Read the model definition and answer for the solid it produces. Units are mm, in the model's axes. Face numbers are marked on the shaded views. Round coordinates to 2 decimals unless told otherwise and drop trailing zeros. Write each loop counter-clockwise with the first axis right and the second up, starting at its lowest first coordinate (ties: lowest second). Pieces come first, ordered by that corner, then holes. Notation, with made-up numbers: (59, 88) -> (66, 88) arc R18 ccw to (66, 118) -> close; hole circle Ø4 at (2, -6.75). An arc over 180 degrees is marked (long way). Return JSON: item names as keys, results as strings.
from build123d import *

# Parameters (mm, degrees)
SKETCH1_W           = 80
SKETCH1_H           = 12
BOSS_EXTRUDE1_DEPTH = 8
SKETCH2_R           = 3
SKETCH2_R_2         = 1
CUT_EXTRUDE1_DEPTH  = 42.231056256
FILLET1_R           = 2


with BuildPart() as part:
    # Sketch1 → Boss-Extrude1 (new body)
    with BuildSketch(Plane(origin=(0, 0, 0), x_dir=(1, 0, 0), z_dir=(0, 1, 0))):
        Rectangle(SKETCH1_W, SKETCH1_H)
    extrude(amount=BOSS_EXTRUDE1_DEPTH)

    # Sketch2 → Cut-Extrude1 (cut, through all)
    with BuildSketch(Plane(origin=(0, 8, 0), x_dir=(1, 0, 0), z_dir=(0, 1, 0))):
        with Locations(Location((-32, 0, 0), (0, 0, 270))):
            Circle(SKETCH2_R)
        with Locations(Location((-12, 0, 0), (0, 0, 270))):
            Circle(SKETCH2_R)
        with Locations(Location((21.25, 0, 0), (0, 0, 270))):
            Circle(SKETCH2_R_2)
        with Locations(Location((30.75, 0, 0), (0, 0, 270))):
            Circle(SKETCH2_R_2)
    extrude(amount=-CUT_EXTRUDE1_DEPTH, mode=Mode.SUBTRACT)

    # Fillet1
    fillet1_edges = [part.edges().sort_by_distance(p)[0] for p in [
        (40, 4, 6),
        (-40, 4, 6),
        (-40, 4, -6),
        (40, 4, -6),
    ]]
    fillet(fillet1_edges, radius=FILLET1_R)


solid = part.part
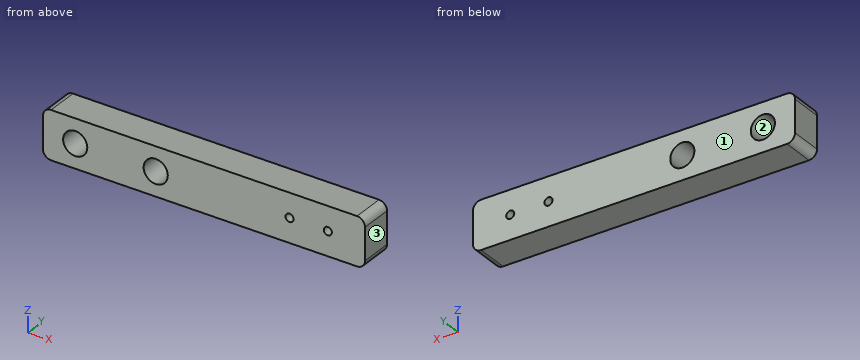
Item 1: Section C-C (z = 0) is taken. Give the vertices of the cut face in (x, y).
Worked answers:
{"outline": "(-40, 0) -> (-35, 0) -> (-35, 8) -> (-40, 8) -> close; (-29, 0) -> (-15, 0) -> (-15, 8) -> (-29, 8) -> close; (-9, 0) -> (20.25, 0) -> (20.25, 8) -> (-9, 8) -> close; (22.25, 0) -> (29.75, 0) -> (29.75, 8) -> (22.25, 8) -> close; (31.75, 0) -> (40, 0) -> (40, 8) -> (31.75, 8) -> close"}
Item 2: Section A-A (x = -32) is taken. Give the vertices of the cut face in (y, z).
Worked answers:
{"outline": "(0, -6) -> (8, -6) -> (8, -3) -> (0, -3) -> close; (0, 3) -> (8, 3) -> (8, 6) -> (0, 6) -> close"}
Item 3: Section B-B (y = 4.5) is taken. Give the vertices of the cut face in (x, z).
Worked answers:
{"outline": "(-40, -4) arc R2 ccw to (-38, -6) -> (38, -6) arc R2 ccw to (40, -4) -> (40, 4) arc R2 ccw to (38, 6) -> (-38, 6) arc R2 ccw to (-40, 4) -> close; hole circle Ø6 at (-32, 0); hole circle Ø6 at (-12, 0); hole circle Ø2 at (21.25, 0); hole circle Ø2 at (30.75, 0)"}
Item 4: A flat-ended cylindrical pin translates along its axis: pin 1 (1.2 mm diameter, centred on x = 30.75, z = 0, fed in from -Y). Find the tip coordinate at first contact, or state that the pin passes through.
Worked answers:
{"pin 1": "passes through"}
Item 5: Section D-D (x = 30.75) is taken. Give the vertices of the cut face in (y, z), then the cut area to 3 significant figures.
Worked answers:
{"outline": "(0, -6) -> (8, -6) -> (8, -1) -> (0, -1) -> close; (0, 1) -> (8, 1) -> (8, 6) -> (0, 6) -> close", "area": "80.0 mm2"}
Item 6: For a pull along X with two mould halves and no side action, classify the marked faces 1, 2 and 3 as released by +X, released by -X, zero draft, split by the parting line, or undercut.
Worked answers:
{"face 1": "zero draft", "face 2": "undercut", "face 3": "released by +X"}
Item 7: Straight lines are drawn through the part: L1, parallel to X at y = 2.75, z = 0; L2, parallel to X at y = 4, z = 2.5; L3, parallel to X at y = 3.5, z = -2.25. For each, find the intervals that lie inside material, in ascending order. Write a range as [from, to].
Worked answers:
{"L1": "x = [-40, -35], [-29, -15], [-9, 20.25], [22.25, 29.75], [31.75, 40]", "L2": "x = [-40, -33.66], [-30.34, -13.66], [-10.34, 40]", "L3": "x = [-40, -33.98], [-30.02, -13.98], [-10.02, 40]"}
